from build123d import *

# Parameters (mm, degrees)
SKETCH1_W           = 185
SKETCH1_H           = 140
BOSS_EXTRUDE1_DEPTH = 70
SHELL1_T            = -5
BOSS_EXTRUDE2_START = 50
SKETCH2_W           = 10
SKETCH2_H           = 130
BOSS_EXTRUDE2_DEPTH = 5
SKETCH3_W           = 10
SKETCH3_H           = 3
BOSS_EXTRUDE6_DEPTH = 5
SKETCH5_W           = 8
SKETCH5_H           = 16
CUT_EXTRUDE1_DEPTH  = 5
SKETCH6_W           = 5
SKETCH6_H           = 5
BOSS_EXTRUDE7_DEPTH = 5


with BuildPart() as part:
    # Sketch1 → Boss-Extrude1 (new body)
    with BuildSketch(Plane.XY):
        Rectangle(SKETCH1_W, SKETCH1_H)
    extrude(amount=BOSS_EXTRUDE1_DEPTH)

    # Shell1
    shell1_openings = [part.faces().sort_by_distance(p)[0] for p in [
        (0, 0, 70),
    ]]
    offset(amount=SHELL1_T, openings=shell1_openings, kind=Kind.INTERSECTION)

    # Sketch2 → Boss-Extrude2 (add)
    with BuildSketch(Plane.XY.offset(5).offset(BOSS_EXTRUDE2_START)):
        with Locations((-72.5, 0)):
            Rectangle(SKETCH2_W, SKETCH2_H)
        with Locations((-42.5, 0)):
            Rectangle(SKETCH2_W, SKETCH2_H)
    extrude(amount=BOSS_EXTRUDE2_DEPTH)

    # Sketch3 → Boss-Extrude6 (add)
    with BuildSketch(Plane.XY.offset(60)):
        Polygon((-47.5, 20), (-27.5, 20), (-27.5, 15), (-24.5, 15), (-24.5, 23), (-47.5, 23), align=None)
        Polygon((-47.5, -20), (-27.5, -20), (-27.5, -15), (-24.5, -15), (-24.5, -23), (-47.5, -23), align=None)
        with Locations((-72.5, 21.5)):
            Rectangle(SKETCH3_W, SKETCH3_H)
        with Locations((-72.5, -21.5)):
            Rectangle(SKETCH3_W, SKETCH3_H)
    extrude(amount=BOSS_EXTRUDE6_DEPTH)

    # Sketch5 → Cut-Extrude1 (cut)
    with BuildSketch(Plane(origin=(92.5, 0, 0), x_dir=(0, 0, -1), z_dir=(1, 0, 0))):
        with Locations((-9, 0)):
            Rectangle(SKETCH5_W, SKETCH5_H)
    extrude(amount=-CUT_EXTRUDE1_DEPTH, mode=Mode.SUBTRACT)

    # Sketch6 → Boss-Extrude7 (add)
    with BuildSketch(Plane.XY.offset(70)):
        with Locations((-90, 67.5)):
            Rectangle(SKETCH6_W, SKETCH6_H)
        with Locations((-90, -67.5)):
            Rectangle(SKETCH6_W, SKETCH6_H)
        with Locations((90, -67.5)):
            Rectangle(SKETCH6_W, SKETCH6_H)
        with Locations((90, 67.5)):
            Rectangle(SKETCH6_W, SKETCH6_H)
    extrude(amount=BOSS_EXTRUDE7_DEPTH)


solid = part.part
Read the model definition and answer for the solid it produces. Units are mm, in the model's axes. A direction names the side the tool comes from. Coordinates: 2 decimals unless noted, no trailing zeros. Order: outer loops, then holes, each group sorted by start corner. A loop starts at its lowest first (then second) coordinate and runs counter-clockwise, first axis right, second up. Notation, with made-up numbers: (-19.5, 20.25) -> (-14.5, 20.25) arc R21 cw to (-14.5, 32.25) -> close; hole circle Ø8 at (51.25, 74). An arc over 180 degrees is marked (long way). Answer as a JSON object with one key per item and string values.
1) A cutting plane is placed at D-D, the plane x = 42. Determine the outline of the cut face in (y, z).
Model answer:
{"outline": "(-70, 0) -> (70, 0) -> (70, 70) -> (65, 70) -> (65, 5) -> (-65, 5) -> (-65, 70) -> (-70, 70) -> close"}
2) Each of these flat-tipped pins is pushed along its axis until it touches: pin 1 (2.5 mm diameter, centred on x = -34, y = 17.5, fed in from -Z); pin 2 (6 mm diameter, centred on x = -33.5, y = -24, fed in from +Z); pin 3 (4 mm diameter, centred on x = 89, y = -21.5, fed in from +Z); pin 4 (8 mm diameter, centred on x = -74, y = 37, fed in from +Z). Where does it stop, or does it pass through?
Model answer:
{"pin 1": "stops at z = 0", "pin 2": "stops at z = 65", "pin 3": "stops at z = 70", "pin 4": "stops at z = 60"}
3) A cutting plane is placed at B-B, the plane z = 67.5. Determine the outline of the cut face in (x, y), plus the area to 3 significant figures.
Model answer:
{"outline": "(-92.5, -70) -> (92.5, -70) -> (92.5, 70) -> (-92.5, 70) -> close; hole (-87.5, -65) -> (87.5, -65) -> (87.5, 65) -> (-87.5, 65) -> close", "area": "3,150 mm²"}
4) A tool of negligible diameter and unlimited length cuts with its end or side. For faces 3 (the face through (-29, -21, 60)), 4 (the face through (-73, 23, 62)), 5 (the face through (90, 1, 70)), 6 (the face through (-87.5, 67, 72)), from which of +Z, -Z, +X, -X, +Y, -Y can it reach the whole face along a straight path? Write none if from no direction.
Model answer:
{"face 3": "none", "face 4": "+Z", "face 5": "+Z, +X, -X", "face 6": "+Z, +Y, -Y"}
5) Consider line 1 along X through (y, z) = (-12, 58.5); line 2 along X through (y, z) = (39, 65.5); line 3 along Y through (x, z) = (66, 34). Determine where each line is inside the solid, lowest interval first. Write a range as from..to.
Model answer:
{"line 1": "x = -92.5..-87.5, -77.5..-67.5, -47.5..-37.5, 87.5..92.5", "line 2": "x = -92.5..-87.5, 87.5..92.5", "line 3": "y = -70..-65, 65..70"}
6) The mould has two halves that part along Y. Classify faces 1 (the face through (-87.5, -68, 72)), 2 (the face through (-90, 65, 72)): released by +Y, released by -Y, zero draft, split by the parting line, or undercut.
Model answer:
{"face 1": "zero draft", "face 2": "undercut"}
7) A cutting plane is placed at C-C, the plane x = -40.5. Determine the outline of the cut face in (y, z).
Model answer:
{"outline": "(-70, 0) -> (70, 0) -> (70, 70) -> (65, 70) -> (65, 60) -> (23, 60) -> (23, 65) -> (20, 65) -> (20, 60) -> (-20, 60) -> (-20, 65) -> (-23, 65) -> (-23, 60) -> (-65, 60) -> (-65, 70) -> (-70, 70) -> close; hole (-65, 5) -> (65, 5) -> (65, 55) -> (-65, 55) -> close"}
8) A cutting plane is placed at A-A, the plane y = 32. Determine the outline of the cut face in (x, z), plus the area to 4 significant figures.
Model answer:
{"outline": "(-92.5, 0) -> (92.5, 0) -> (92.5, 70) -> (87.5, 70) -> (87.5, 5) -> (-87.5, 5) -> (-87.5, 70) -> (-92.5, 70) -> close; (-77.5, 55) -> (-67.5, 55) -> (-67.5, 60) -> (-77.5, 60) -> close; (-47.5, 55) -> (-37.5, 55) -> (-37.5, 60) -> (-47.5, 60) -> close", "area": "1,675 mm²"}
